Part model, mm, in its own coordinate system. Give positions to 0.01 mm unless a question says otherwise; leave off trailing zeros. Write each loop counter-clockwise with the first axis right and the second up, starting at its lowest first coordinate (ties: lowest second). Pieces come first, ordered by that corner, then holes.
from build123d import *

# Parameters (mm, degrees)
SKETCH2_R           = 2.05
BOSS_EXTRUDE1_DEPTH = 3
BOSS_EXTRUDE2_DEPTH = 3
FILLET1_R           = 1


with BuildPart() as part:
    # Sketch2 → Boss-Extrude1 (new body)
    # profile 1 of 2: a face of its own
    with BuildSketch(Plane(origin=(0, 0, 0), x_dir=(-1, 0, 0), z_dir=(0, 0, 1))):
        with BuildLine():
            Line((125, 0), (-125, 0))
            ThreePointArc((-125, 0), (-135.606601718, -4.393398282), (-140, -15))
            Line((-140, -15), (-140, -172.349939952))
            ThreePointArc((-140, -172.349939952), (-138.469261815, -178.951378141), (-134.189468511, -184.205473195))
            Line((-134.189468511, -184.205473195), (134.189468511, -184.205473195))
            ThreePointArc((134.189468511, -184.205473195), (138.469261815, -178.951378141), (140, -172.349939952))
            Line((140, -172.349939952), (140, -15))
            ThreePointArc((140, -15), (135.606601718, -4.393398282), (125, 0))
        make_face()
        with Locations(Location((132, -179.349939952, 0), (0, 0, 180))):
            Circle(SKETCH2_R, mode=Mode.SUBTRACT)
        with Locations(Location((132, -8, 0), (0, 0, 180))):
            Circle(SKETCH2_R, mode=Mode.SUBTRACT)
        with Locations(Location((-132, -8, 0), (0, 0, 180))):
            Circle(SKETCH2_R, mode=Mode.SUBTRACT)
        with Locations(Location((-132, -179.349939952, 0), (0, 0, 180))):
            Circle(SKETCH2_R, mode=Mode.SUBTRACT)
        with BuildLine():
            ThreePointArc((127, -10), (126.414213562, -8.585786438), (125, -8))
            Line((125, -8), (-125, -8))
            ThreePointArc((-125, -8), (-126.414213562, -8.585786438), (-127, -10))
            Line((-127, -10), (-127, -177.349939952))
            ThreePointArc((-127, -177.349939952), (-126.414213562, -178.764153514), (-125, -179.349939952))
            Line((-125, -179.349939952), (125, -179.349939952))
            ThreePointArc((125, -179.349939952), (126.414213562, -178.764153514), (127, -177.349939952))
            Line((127, -177.349939952), (127, -10))
        make_face(mode=Mode.SUBTRACT)
    # profile 2 of 2: a face of its own
    with BuildSketch(Plane(origin=(0, 0, 0), x_dir=(-1, 0, 0), z_dir=(0, 0, 1))):
        with BuildLine():
            Line((127, -10), (127, -177.349939952))
            ThreePointArc((127, -177.349939952), (126.414213562, -178.764153514), (125, -179.349939952))
            Line((125, -179.349939952), (-125, -179.349939952))
            ThreePointArc((-125, -179.349939952), (-126.414213562, -178.764153514), (-127, -177.349939952))
            Line((-127, -177.349939952), (-127, -10))
            ThreePointArc((-127, -10), (-126.414213562, -8.585786438), (-125, -8))
            Line((-125, -8), (125, -8))
            ThreePointArc((125, -8), (126.414213562, -8.585786438), (127, -10))
        make_face()
    extrude(amount=BOSS_EXTRUDE1_DEPTH)

    # Sketch3 → Boss-Extrude2 (add)
    with BuildSketch(Plane(origin=(0, 0, 0), x_dir=(-1, 0, 0), z_dir=(0, 0, -1))):
        with BuildLine():
            Line((-126.6, 177.349939952), (-126.6, 10))
            ThreePointArc((-126.6, 10), (-126.13137085, 8.86862915), (-125, 8.4))
            Line((-125, 8.4), (125, 8.4))
            ThreePointArc((125, 8.4), (126.13137085, 8.86862915), (126.6, 10))
            Line((126.6, 10), (126.6, 177.349939952))
            ThreePointArc((126.6, 177.349939952), (126.13137085, 178.481310802), (125, 178.949939952))
            Line((125, 178.949939952), (-125, 178.949939952))
            ThreePointArc((-125, 178.949939952), (-126.13137085, 178.481310802), (-126.6, 177.349939952))
        make_face()
    extrude(amount=BOSS_EXTRUDE2_DEPTH)

    # Fillet1
    fillet1_edges = [part.edges().sort_by_distance(p)[0] for p in [
        (-134.05, 8, 3),
        (129.95, 8, 3),
        (129.95, 179.349939952, 3),
        (-134.05, 179.349939952, 3),
    ]]
    fillet(fillet1_edges, radius=FILLET1_R)


solid = part.part
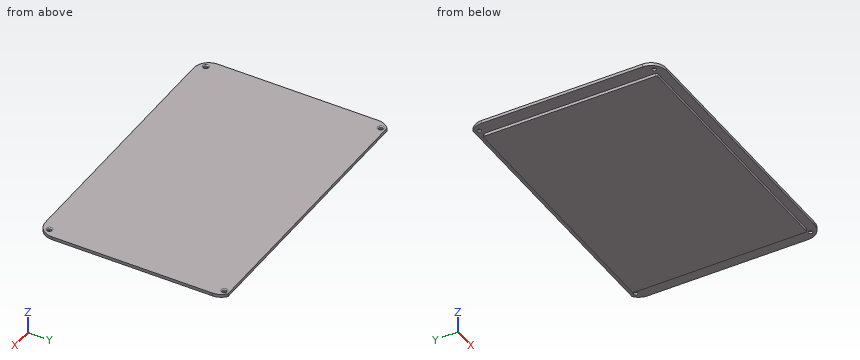
1) Saw through at A-A (y = 135). Write the cut outline in (x, z).
Check result:
outline: (-140, 0) - (-126.6, 0) - (-126.6, -3) - (126.6, -3) - (126.6, 0) - (140, 0) - (140, 3) - (-140, 3) - close
2) Drill centre lines: L1, parallel to Y at x = 132, z = 0.6; L2, parallel to Y at x = 95, z = -0.65; L3, parallel to X at y = 176.5, z = -0.4. Where is each one in solid material? Low to high.
Check result:
L1: y = 1.73 to 5.95, 10.05 to 177.3, 181.4 to 184.21
L2: y = 8.4 to 178.95
L3: x = -126.6 to 126.6
3) Flat gauge pins, fed straight in: P1, Ø4.5, axis at x = 132, y = 8, coming from the +Z side; P2, Ø1, axis at y = 85.5, z = -1.5, coming from the +X side; P3, Ø2.5, axis at x = 56, z = -2, coming from the -Y side. Where does each tip first touch, or does it go through?
Check result:
P1: stops at z = 2.6
P2: stops at x = 126.6
P3: stops at y = 8.4
4) Saw through at B-B (x = 107.5). Write the cut outline in (y, z).
Check result:
outline: (0, 0) - (8.4, 0) - (8.4, -3) - (178.95, -3) - (178.95, 0) - (184.21, 0) - (184.21, 3) - (0, 3) - close
